```python
from build123d import *

# Parameters (mm, degrees)
SKETCH_1_W          = 96
SKETCH_1_H          = 20
EXTRUDE_1_DEPTH     = 10
SKETCH_2_R          = 5
CUT_EXTRUDE_1_DEPTH = 5
FILLET_1_R          = 10
SKETCH_3_R          = 3.1
CUT_EXTRUDE_2_DEPTH = 5
CHAMFER_1_SIZE      = 1
SKETCH_4_W          = 50
SKETCH_4_H          = 20
EXTRUDE_2_DEPTH     = 50.5
CUT_EXTRUDE_START   = -20
CUT_EXTRUDE_4_DEPTH = 20
SKETCH_7_R          = 17.6
CUT_EXTRUDE_5_DEPTH = 16
SKETCH_8_R          = 15
CUT_EXTRUDE_6_DEPTH = 16
CHAMFER_3_SIZE      = 2
FILLET_3_R          = 5
CHAMFER_5_SIZE      = 2
SKETCH_9_W          = 30
SKETCH_9_H          = 15
CUT_EXTRUDE_7_DEPTH = 80.776249598
FILLET_4_R          = 5
CHAMFER_6_SIZE      = 2


# Read off the part's stored shape, not the designer's step: 切除-拉伸4
with BuildPart() as part:
    # 草图1 → 凸台-拉伸1 (new body)
    with BuildSketch(Plane(origin=(0, 0, 0), x_dir=(1, 0, 0), z_dir=(0, 1, 0))):
        Rectangle(SKETCH_1_W, SKETCH_1_H)
    extrude(amount=EXTRUDE_1_DEPTH)

    # 草图2 → 切除-拉伸1 (cut)
    with BuildSketch(Plane(origin=(0, 10, 0), x_dir=(1, 0, 0), z_dir=(0, 1, 0))):
        with Locations(Location((-38, 0, 0), (0, 0, 270))):
            Circle(SKETCH_2_R)
        with Locations(Location((38, 0, 0), (0, 0, 90))):
            Circle(SKETCH_2_R)
    extrude(amount=-CUT_EXTRUDE_1_DEPTH, mode=Mode.SUBTRACT)

    # 圆角1
    fillet_1_edges = [part.edges().sort_by_distance(p)[0] for p in [
        (48, 5, -10),
        (48, 5, 10),
        (-48, 5, 10),
        (-48, 5, -10),
    ]]
    fillet(fillet_1_edges, radius=FILLET_1_R - 0.0001)  # a hair under: the kernel refuses the full size

    # 草图3 → 切除-拉伸2 (cut)
    with BuildSketch(Plane(origin=(0, 5, 0), x_dir=(1, 0, 0), z_dir=(0, 1, 0))):
        with Locations(Location((-38, 0, 0), (0, 0, 270))):
            Circle(SKETCH_3_R)
        with Locations(Location((38, 0, 0), (0, 0, 270))):
            Circle(SKETCH_3_R)
    extrude(amount=-CUT_EXTRUDE_2_DEPTH, mode=Mode.SUBTRACT)

    # 倒角1
    chamfer_1_edges = [part.edges().sort_by_distance(p)[0] for p in [
        (-38, 0, -3.1),
        (38, 0, -3.1),
    ]]
    chamfer(chamfer_1_edges, length=CHAMFER_1_SIZE)

    # 草图4 → 凸台-拉伸2 (add)
    with BuildSketch(Plane(origin=(0, 10, 0), x_dir=(1, 0, 0), z_dir=(0, 1, 0))):
        Rectangle(SKETCH_4_W, SKETCH_4_H)
    extrude(amount=EXTRUDE_2_DEPTH)

    # 切除-拉伸4 outline → 切除-拉伸4 (cut)
    with BuildSketch(Plane.XY.offset(10).offset(CUT_EXTRUDE_START)):
        with BuildLine():
            Line((-25, 60.5), (-25, 35.5))
            ThreePointArc((-25, 35.5), (-17.677669559, 53.1776695), (-8.4e-08, 60.5))
            Line((-8.4e-08, 60.5), (-25, 60.5))
        make_face()
        with BuildLine():
            Line((25, 60.5), (-8.4e-08, 60.5))
            ThreePointArc((-8.4e-08, 60.5), (17.6776695, 53.177669559), (25, 35.5))
            Line((25, 35.5), (25, 60.5))
        make_face()
    extrude(amount=CUT_EXTRUDE_4_DEPTH, mode=Mode.SUBTRACT)

    # 草图7 → 切除-拉伸5 (cut)
    with BuildSketch(Plane.XY.offset(10)):
        with Locations((0, 35.5)):
            Circle(SKETCH_7_R)
    extrude(amount=-CUT_EXTRUDE_5_DEPTH, mode=Mode.SUBTRACT)

    # 草图8 → 切除-拉伸6 (cut)
    with BuildSketch(Plane.XY.offset(-6)):
        with Locations((0, 35.5)):
            Circle(SKETCH_8_R)
    extrude(amount=-CUT_EXTRUDE_6_DEPTH, mode=Mode.SUBTRACT)

    # 倒角3
    chamfer_3_edges = [part.edges().sort_by_distance(p)[0] for p in [
        (-17.6, 35.5, 10),
    ]]
    chamfer(chamfer_3_edges, length=CHAMFER_3_SIZE)

    # 圆角3
    fillet_3_edges = [part.edges().sort_by_distance(p)[0] for p in [
        (25, 10, 0),
        (-25, 10, 0),
    ]]
    fillet(fillet_3_edges, radius=FILLET_3_R)

    # 倒角5
    chamfer_5_edges = [part.edges().sort_by_distance(p)[0] for p in [
        (34.00005, 10, 10),
        (34.00005, 10, -10),
        (26.464466094, 11.464466094, -10),
        (26.464466094, 11.464466094, 10),
        (-26.464466094, 11.464466094, 10),
        (-26.464466094, 11.464466094, -10),
        (-34.00005, 10, -10),
        (-34.00005, 10, 10),
        (-45.071097101, 10, -7.071097101),
        (-45.071097101, 10, 7.071097101),
        (45.071097101, 10, 7.071097101),
        (45.071097101, 10, -7.071097101),
        (-25, 25.25, 10),
        (-25, 25.25, -10),
        (25, 25.25, -10),
        (25, 25.25, 10),
        (17.6776695, 53.177669559, -10),
        (17.6776695, 53.177669559, 10),
    ]]
    chamfer(chamfer_5_edges, length=CHAMFER_5_SIZE)

    # 草图9 → 切除-拉伸7 (cut, through all)
    with BuildSketch(Plane.XY.offset(10)):
        Rectangle(SKETCH_9_W, SKETCH_9_H)
    extrude(amount=-CUT_EXTRUDE_7_DEPTH, mode=Mode.SUBTRACT)

    # 圆角4
    fillet_4_edges = [part.edges().sort_by_distance(p)[0] for p in [
        (15, 7.5, 0),
        (-15, 7.5, 0),
    ]]
    fillet(fillet_4_edges, radius=FILLET_4_R)

    # 倒角6
    chamfer_6_edges = [part.edges().sort_by_distance(p)[0] for p in [
        (15, 1.25, -10),
        (15, 1.25, 10),
        (0, 7.5, 10),
        (0, 7.5, -10),
        (-15, 1.25, -10),
        (-15, 1.25, 10),
        (13.535533906, 6.035533906, 10),
        (13.535533906, 6.035533906, -10),
        (-13.535533906, 6.035533906, 10),
        (-13.535533906, 6.035533906, -10),
    ]]
    chamfer(chamfer_6_edges, length=CHAMFER_6_SIZE)


solid = part.part
```
Check sheet for the modelled part. Datum: model origin and axes. Units: mm. A direction names the side the tool comes from. Round coordinates to 2 decimals unless told otherwise and drop trailing zeros. One line per question, with ' | ' between items. Start each with the question number.
1. Sectioned sample at A-A, the plane z = -1.75. Count the separate pieces of the cut face and the enclosed holes in it, then the cut area to 3 significant figures.
2. Set-up check for faces 4 (the face through (-33.043, 7.535, -0.651)), 5 (the face through (34, 9, -9)), 6 (the face through (16, 1, 9)), 7 (the face through (15, 1, 0)), 8 (the face through (-3.82, 18.32, 1.1)): record each of +Z, -Z, +X, -X, +Y, -Y from which the full face is reachable in a straight line by a thin tool's end or side.
3. Release check for a two-part mould opening along Z. For faces 1 (the face through (41.074, 3.028, -0.404)), 2 (the face through (14.12, 6.531, 8.764)), 3 (the face through (27, 11, 0)) record: +Z half, -Z half, draft (parallel to the pull), parting line (faces both ways), or undercut.
4. Depth check by flat-ended pin: pin 1 (0.8 mm diameter, centred on y = 1, z = -2.5, fed in from +X); pin 2 (1 mm diameter, centred on x = -14.5, z = -3, fed in from +Y); pin 3 (5 mm diameter, centred on x = 2, z = 1, fed in from -Y). Enter the tip coordinate at first touch or a pass-through.
5. Scan lines: line 1 along Y through (x, z) = (0, -2.75); line 2 along Y through (x, z) = (0, -7); line 3 along X through (y, z) = (4.05, 0). Record each from-to range of solid material in increasing order. Write a range as from..to.
Taken from the geometry:
1) separate pieces: 3 | enclosed holes: 1 | area: 1,890 mm^2
2) face 4: +Y | face 5: -Z, +X, +Y | face 6: +Z, -Y | face 7: +Z, -Z, -Y | face 8: +Z
3) face 1: undercut | face 2: +Z half | face 3: draft
4) pin 1: stops at x = 47.78 | pin 2: stops at y = 56.21 | pin 3: stops at y = 7.5
5) line 1: y = 7.5..17.9, 53.1..60.5 | line 2: y = 7.5..20.5, 50.5..60.5 | line 3: x = -48..-41.1, -34.9..-14.75, 14.75..34.9, 41.1..48
